```python
from build123d import *

# Parameters (mm, degrees)
SKETCH_1_R          = 1.075
EXTRUDE_1_DEPTH     = 7
SKETCH_3_R          = 2.55
CUT_EXTRUDE_1_DEPTH = 2.4
SKETCH_4_R          = 3.1
CUT_EXTRUDE_3_DEPTH = 0.8


with BuildPart() as part:
    # 草图1 → 凸台-拉伸1 (new body)
    with BuildSketch(Plane(origin=(0, 0, 0), x_dir=(1, 0, 0), z_dir=(0, 1, 0))):
        with BuildLine():
            Line((0, 0), (47.5, 0))
            ThreePointArc((47.5, 0), (51.5, -4), (47.5, -8))
            Line((47.5, -8), (0, -8))
            ThreePointArc((0, -8), (-4, -4), (0, 0))
        make_face()
        with Locations((0, -4)):
            Circle(SKETCH_1_R, mode=Mode.SUBTRACT)
        with Locations((19, -4)):
            Circle(SKETCH_1_R, mode=Mode.SUBTRACT)
        with Locations((47.5, -4)):
            Circle(SKETCH_1_R, mode=Mode.SUBTRACT)
    extrude(amount=EXTRUDE_1_DEPTH)

    # 草图3 → 切除-拉伸1 (cut)
    with BuildSketch(Plane(origin=(0, 7, 0), x_dir=(1, 0, 0), z_dir=(0, 1, 0))):
        with Locations((0, -4)):
            Circle(SKETCH_3_R)
        with Locations((19, -4)):
            Circle(SKETCH_3_R)
        with Locations((47.5, -4)):
            Circle(SKETCH_3_R)
    extrude(amount=-CUT_EXTRUDE_1_DEPTH, mode=Mode.SUBTRACT)

    # 草图4 → 切除-拉伸3 (cut)
    with BuildSketch(Plane(origin=(0, 7, 0), x_dir=(1, 0, 0), z_dir=(0, 1, 0))):
        with Locations((0, -4)):
            Circle(SKETCH_4_R)
        with Locations((19, -4)):
            Circle(SKETCH_4_R)
        with Locations((47.5, -4)):
            Circle(SKETCH_4_R)
    extrude(amount=-CUT_EXTRUDE_3_DEPTH, mode=Mode.SUBTRACT)


solid = part.part
```
Design review of the part built by this model. Coordinates are the model's own, in mm. A direction names the side the tool comes from. Coordinates: 2 decimals unless noted, no trailing zeros. Order: outer loops, then holes, each group sorted by start corner. A loop starts at its lowest first (then second) coordinate and runs counter-clockwise, first axis right, second up. Notation, with made-up numbers: (67.5, 47.25) -> (101.5, 47.25) arc R24 ccw to (101.5, 66.25) -> close; hole circle Ø2 at (52.5, 34). An arc over 180 degrees is marked (long way). One line per item, written item: value. Start each with the question number.
Q1. Insertion check: pin 1 Ø4 at (x, z) = (1, 3) entering from +Y; pin 2 Ø1.5 at (x, z) = (46.5, 3) entering from +Y. Each pin has a flat end and moves straight along its axis. Give the tip position at first contact, or say it passes through.
Q2. Tool access review of faces 1 (the cylindrical face through (46.426, 2.268, 3.953)), 2 (the cylindrical face through (18.328, 6.606, 7.026)): name each direction out of +Z, -Z, +X, -X, +Y, -Y from which nothing blocks a thin tool from reaching the whole face with its end or side.
Q3. For probe 1 along X at (y, z) = (5.45, 4); probe 2 along X at (y, z) = (6.6, 4); probe 3 along Z at (x, y) = (19, 2.65) (3 decimals), list the stretches that pass through material, from the lowest coordinate up.
Q4. Take a section at B-B, the plane y = 1. State the section outline as (x, z) points (3 decimals), then the cut area to 3 significant figures.
Q5. Take a section at D-D, the plane y = 5.25. State the section outline as (x, z) points.
Q6. Take a section at C-C, the plane z = 4. Give the number of separate pieces and of enclosed holes in the cut face, then the cut area to 3 significant figures.
Q7. Take a section at A-A, the plane x = 19. State the section outline as (y, z) points (3 decimals).
Q8. Mouldability with a two-part tool opening along X and no side actions: class faces 3 (the flat face through (24, 0, 4)), 4 (the cylindrical face through (-4, 3, 4)), 5 (the cylindrical face through (20.025, 2.268, 3.677)) as pulls with the +X half, pulls with the -X half, needs draft (parallel to the pull), parting line crosses it, or undercut.
Values follow:
1. pin 1: stops at y = 7
1. pin 2: stops at y = 4.6
2. face 1: +Y, -Y
2. face 2: +Y
3. probe 1: x = -4 to -2.55, 2.55 to 16.45, 21.55 to 44.95, 50.05 to 51.5
3. probe 2: x = -4 to -3.1, 3.1 to 15.9, 22.1 to 44.4, 50.6 to 51.5
3. probe 3: z = 0 to 2.925, 5.075 to 8
4. outline: (0, 0) -> (47.5, 0) arc R4 ccw to (47.5, 8) -> (0, 8) arc R4 ccw to start; hole circle Ø2.15 at (0, 4); hole circle Ø2.15 at (19, 4); hole circle Ø2.15 at (47.5, 4)
4. area: 419 mm2
5. outline: (0, 0) -> (47.5, 0) arc R4 ccw to (47.5, 8) -> (0, 8) arc R4 ccw to start; hole circle Ø5.1 at (0, 4); hole circle Ø5.1 at (19, 4); hole circle Ø5.1 at (47.5, 4)
6. separate pieces: 4
6. enclosed holes: 0
6. area: 319 mm2
7. outline: (0, 0) -> (7, 0) -> (7, 0.9) -> (6.2, 0.9) -> (6.2, 1.45) -> (4.6, 1.45) -> (4.6, 2.925) -> (0, 2.925) -> close; (0, 5.075) -> (4.6, 5.075) -> (4.6, 6.55) -> (6.2, 6.55) -> (6.2, 7.1) -> (7, 7.1) -> (7, 8) -> (0, 8) -> close
8. face 3: needs draft
8. face 4: pulls with the -X half
8. face 5: undercut
